```python
from build123d import *

# Parameters (mm, degrees)
SKETCH1_R           = 32.5
BOSS_EXTRUDE1_DEPTH = 60.791802
SKETCH2_R           = 27.69421809
CUT_EXTRUDE1_DEPTH  = 77.211174971
CHAMFER1_SIZE       = 2.267082


with BuildPart() as part:
    # Sketch1 → Boss-Extrude1 (new body)
    with BuildSketch(Plane(origin=(0, 0, 0), x_dir=(1, 0, 0), z_dir=(0, 1, 0))):
        with Locations(Location((0, 0, 0), (0, 0, 270))):
            Circle(SKETCH1_R)
    extrude(amount=BOSS_EXTRUDE1_DEPTH)

    # Sketch2 → Cut-Extrude1 (cut, through all)
    with BuildSketch(Plane(origin=(0, 0, 0), x_dir=(1, 0, 0), z_dir=(0, 1, 0))):
        with Locations(Location((0, 0, 0), (0, 0, 270))):
            Circle(SKETCH2_R)
    extrude(amount=CUT_EXTRUDE1_DEPTH, mode=Mode.SUBTRACT)

    # Chamfer1
    chamfer1_edges = [part.edges().sort_by_distance(p)[0] for p in [
        (0, 0, -32.5),
        (0, 60.791802, -32.5),
        (0, 0, -27.69421809),
        (0, 60.791802, -27.69421809),
    ]]
    chamfer(chamfer1_edges, length=CHAMFER1_SIZE)


solid = part.part
```
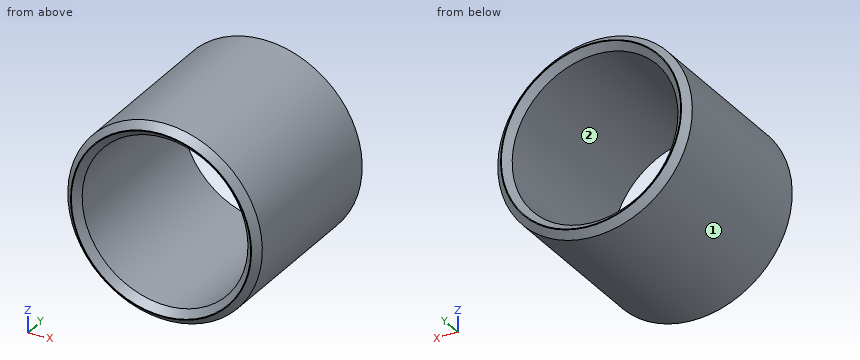
For this review, take the finished solid that the model builds, in its own axes (mm). Face numbers are marked on the shaded views. Coordinates: 2 decimals unless noted, no trailing zeros. Loops run counter-clockwise (first coordinate to the right, second up) from the corner with the lowest first, then second, coordinate; pieces in that order, holes last. Notation, with made-up numbers: (69.25, -7.75) -> (84.25, -7.75) arc R35 cw to (84.25, 25.25) -> close; hole circle Ø11 at (-14.75, 70). An arc over 180 degrees is marked (long way). Return JSON: item names as keys, results as strings. Group by question number.
(1) Consider section B-B, the plane z = 0. Give the boundary of the cut face in (x, y).
(2) For pin 1 Ø1.5 at (y, z) = (23, -5.5) entering from +X; pin 2 Ø12 at (y, z) = (51, -8.5) entering from +X; pin 3 Ø1.5 at (x, y) = (-6, 7.5) entering from -Z, all flat-tipped, find the tip position at first contact; note any pin that passes through.
(3) Consider section C-C, the plane y = 18. Give the boundary of the cut face in (x, z), plus the area to 3 significant figures.
(4) To check wall thickness, follow L1, parallel to X at y = 21, z = 0; L2, parallel to Z at x = 5, y = 42; L3, parallel to Z at x = -11, y = 7.5. State the ranges of each line that lie inside material, in increasing order.
(5) Consider section A-A, the plane x = 0. Give the boundary of the cut face in (y, z), plus the area to 3 significant figures.
(6) Mouldability with a two-part tool opening along X and no side actions: class the marked faces 1 and 2 as pulls with the +X half, pulls with the -X half, needs draft (parallel to the pull), parting line crosses it, or undercut.
Results below:
{
 "1": {"outline": "(-32.5, 2.27) -> (-30.23, 0) -> (-29.96, 0) -> (-27.69, 2.27) -> (-27.69, 58.52) -> (-29.96, 60.79) -> (-30.23, 60.79) -> (-32.5, 58.52) -> close; (27.69, 2.27) -> (29.96, 0) -> (30.23, 0) -> (32.5, 2.27) -> (32.5, 58.52) -> (30.23, 60.79) -> (29.96, 60.79) -> (27.69, 58.52) -> close"},
 "2": {"pin 1": "stops at x = 32.15", "pin 2": "stops at x = 32.4", "pin 3": "stops at z = -32.07"},
 "3": {"outline": "circle Ø65 at (0, 0); hole circle Ø55.39 at (0, 0)", "area": "909 mm2"},
 "4": {"L1": "x = -32.5 to -27.69, 27.69 to 32.5", "L2": "z = -32.11 to -27.24, 27.24 to 32.11", "L3": "z = -30.58 to -25.42, 25.42 to 30.58"},
 "5": {"outline": "(0, -30.23) -> (2.27, -32.5) -> (58.52, -32.5) -> (60.79, -30.23) -> (60.79, -29.96) -> (58.52, -27.69) -> (2.27, -27.69) -> (0, -29.96) -> close; (0, 29.96) -> (2.27, 27.69) -> (58.52, 27.69) -> (60.79, 29.96) -> (60.79, 30.23) -> (58.52, 32.5) -> (2.27, 32.5) -> (0, 30.23) -> close", "area": "564 mm2"},
 "6": {"face 1": "parting line crosses it", "face 2": "undercut"}
}
